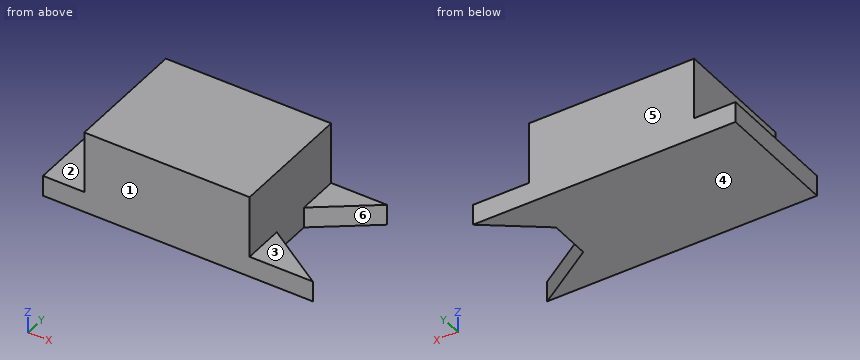
from build123d import *

# Parameters (mm, degrees)
F0_W     = 25.4
F0_H     = 76.2
F1_DEPTH = 12.7
F2_DEPTH = 50.8
F3_DEPTH = 12.7
F4_DEPTH = 12.7


with BuildPart() as f1:
    # F0 (on Top) → F1 (new body)
    with BuildSketch(Plane.XY):
        with Locations((-24.833125, -3.603618)):
            Rectangle(F0_W, F0_H)
    extrude(amount=F1_DEPTH)

    # F0 (on Top) → F2 (join)
    with BuildSketch(Plane.XY):
        Polygon((89.466875, 34.496382), (-12.133125, 34.496382), (-12.133125, -41.703618), (89.466875, -41.703618), (89.466875, -16.303618), (89.466875, 9.096382), align=None)
    extrude(amount=F2_DEPTH)

    # F0 (on Top) → F3 (join)
    with BuildSketch(Plane.XY):
        Polygon((123.831588, 34.496382), (89.466875, 34.496382), (89.466875, 9.096382), align=None)
    extrude(amount=F3_DEPTH)

    # F0 (on Top) → F4 (join)
    with BuildSketch(Plane.XY):
        Polygon((89.466875, -16.303618), (89.466875, -41.703618), (128.313944, -41.703618), align=None)
    extrude(amount=F4_DEPTH)


solid = f1.part
CAD build for the part. Positions are in the model's coordinates, mm. Face numbers are marked on the shaded views. A direction names the side the tool comes from. Round coordinates to 2 decimals unless told otherwise and drop trailing zeros. Write each loop counter-clockwise with the first axis right and the second up, starting at its lowest first coordinate (ties: lowest second). Pieces come first, ordered by that corner, then holes. Notation, with made-up numbers: M 24,-28.75 L 64,-28.75 A24 ccw 64,-11.75 Z; hole C 6,36 d8. An arc over 180 degrees is marked long. Use a Markdown table: item, result. Add a question column.
1. Slice it at D-D on z = 31. Give the cut face in (x, y), then the cut area to 3 significant figures.
2. Drill centre lines: probe 1 along X at (y, z) = (-13.5, 22.5); probe 2 along Z at (x, y) = (-13, 9.5); probe 3 along Y at (x, z) = (96, 9). Where is each one in solid material? Low to high.
3. Flat gauge pins, fed straight in: P1, Ø20.5, axis at x = 107, y = -25, coming from the +Z side; P2, Ø5, axis at y = -21.5, z = 37, coming from the +X side; P3, Ø11.5, axis at y = -16, z = 38.5, coming from the -X side; P4, Ø12, axis at x = -16.5, z = 40, coming from the +Y side. Where does each tip first touch, or does it go through?
4. Slice it at C-C on y = -26.5. Give the cut face in (x, z).
5. Pull direction Y, two halves, no side cores. Call the marked faces 4, 5 and 6: released by +Y, released by -Y, zero draft, split by the parting line, or undercut.
6. Slice it at A-A on y = 22.5. Give the cut face in (x, z).
7. 3-axis set-ups, long thin cutter, end or side, ignore diameter. For the marked faces 1, 2 and 3: which of +Z, -Z, +X, -X, +Y, -Y reach the whole face in a straight line?
8. Slice it at B-B on z = 6. Give the cut face in (x, y), then the cut area to 3 significant figures.
Reply:
| question | item | result |
|---|---|---|
| 1 | outline | M -12.13,-41.7 L 89.47,-41.7 L 89.47,34.5 L -12.13,34.5 Z |
| 1 | area | 7,740 mm^2 |
| 2 | probe 1 | x = -12.13 to 89.47 |
| 2 | probe 2 | z = 0 to 12.7 |
| 2 | probe 3 | y = -41.7 to -20.58, 13.93 to 34.5 |
| 3 | P1 | stops at z = 12.7 |
| 3 | P2 | stops at x = 89.47 |
| 3 | P3 | stops at x = -12.13 |
| 3 | P4 | stops at y = 34.5 |
| 4 | outline | M -37.53,0 L 105.06,0 L 105.06,12.7 L 89.47,12.7 L 89.47,50.8 L -12.13,50.8 L -12.13,12.7 L -37.53,12.7 Z |
| 5 | face 4 | zero draft |
| 5 | face 5 | released by +Y |
| 5 | face 6 | undercut |
| 6 | outline | M -37.53,0 L 107.6,0 L 107.6,12.7 L 89.47,12.7 L 89.47,50.8 L -12.13,50.8 L -12.13,12.7 L -37.53,12.7 Z |
| 7 | face 1 | +Z, -Z, +X, -X, -Y |
| 7 | face 2 | +Z, -X, +Y, -Y |
| 7 | face 3 | +Z, +X, +Y, -Y |
| 8 | outline | M -37.53,-41.7 L 128.31,-41.7 L 89.47,-16.3 L 89.47,9.1 L 123.83,34.5 L -37.53,34.5 Z |
| 8 | area | 10,600 mm^2 |
